from build123d import *

# Parameters (mm, degrees)
ESQUISSE1_R             = 17.5
ESQUISSE1_R_2           = 12.5
BOSS_EXTRU_1_DEPTH      = 65
ESQUISSE3_R             = 2.65
ENL_V_MAT_EXTRU_1_DEPTH = 4
ESQUISSE4_R             = 2
BOSS_EXTRU_2_DEPTH      = 1
BOSS_EXTRU_2_DEPTH_BACK = 2
ENL_V_MAT_EXTRU_2_REACH = 38
ESQUISSE5_R             = 1.05
ENL_V_START             = -3.5
ESQUISSE6_R             = 2.5
ENL_V_MAT_EXTRU_3_DEPTH = 5
CONG_1_R                = 0.5
CHANFREIN1_SIZE         = 0.1
ESQUISSE7_R             = 17.5
BOSS_EXTRU_3_DEPTH      = 5
CHANFREIN2_SIZE         = 2
CHANFREIN3_SIZE         = 1
CHANFREIN3_SIZE2        = 0.577350269


with BuildPart() as part:
    # Esquisse1 → Boss.-Extru.1 (new body, symmetric)
    with BuildSketch(Plane(origin=(0, 0, 0), x_dir=(1, 0, 0), z_dir=(0, 1, 0))):
        Circle(ESQUISSE1_R)
        Circle(ESQUISSE1_R_2, mode=Mode.SUBTRACT)
    extrude(amount=BOSS_EXTRU_1_DEPTH, both=True)

    # Esquisse3 → Enlèv. mat.-Extru.1 (cut)
    with BuildSketch(Plane(origin=(17.5, 0, 0), x_dir=(0, 0, -1), z_dir=(1, 0, 0))):
        Circle(ESQUISSE3_R)
    enl_v_mat_extru_1 = extrude(amount=-ENL_V_MAT_EXTRU_1_DEPTH, mode=Mode.SUBTRACT)

    # Symétrie1: Enlèv. mat.-Extru.1 across plane
    add(enl_v_mat_extru_1.mirror(Plane(origin=(0, 0, 0), x_dir=(0, 0, 1), z_dir=(1, 0, 0))), mode=Mode.SUBTRACT)

    # Esquisse4 → Boss.-Extru.2 (add, two sides)
    with BuildSketch(Plane(origin=(17.5, 0, 0), x_dir=(0, 0, -1), z_dir=(1, 0, 0))) as boss_extru_2_sk:
        with Locations((0, -50)):
            Circle(ESQUISSE4_R)
    extrude(amount=BOSS_EXTRU_2_DEPTH)
    extrude(boss_extru_2_sk.sketch, amount=-BOSS_EXTRU_2_DEPTH_BACK)

    # Esquisse5 → Enlèv. mat.-Extru.2 (cut, up to next)
    with BuildSketch(Plane(origin=(18.5, 0, 0), x_dir=(0, 0, -1), z_dir=(1, 0, 0)), mode=Mode.PRIVATE) as enl_v_mat_extru_2_sk1:
        with Locations((0, -50)):
            Circle(ESQUISSE5_R)
    enl_v_mat_extru_2_tool1 = extrude(enl_v_mat_extru_2_sk1.sketch, amount=-ENL_V_MAT_EXTRU_2_REACH, mode=Mode.PRIVATE) & part.part
    add(enl_v_mat_extru_2_tool1.solids().sort_by_distance((18.5, -50, 0))[0], mode=Mode.SUBTRACT)

    # Esquisse6 → Enlèv. mat.-Extru.3 (cut)
    with BuildSketch(Plane(origin=(18.5, 0, 0), x_dir=(0, 0, -1), z_dir=(1, 0, 0)).offset(ENL_V_START)):
        with Locations((0, -50)):
            Circle(ESQUISSE6_R)
    extrude(amount=-ENL_V_MAT_EXTRU_3_DEPTH, mode=Mode.SUBTRACT)

    # Congé1
    cong_1_edges = [part.edges().sort_by_distance(p)[0] for p in [
        (17.385338651, -50, 2),
    ]]
    fillet(cong_1_edges, radius=CONG_1_R)

    # Chanfrein1
    chanfrein1_edges = [part.edges().sort_by_distance(p)[0] for p in [
        (18.5, -50, 2),
    ]]
    chamfer(chanfrein1_edges, length=CHANFREIN1_SIZE)

    # Esquisse7 → Boss.-Extru.3 (add)
    with BuildSketch(Plane(origin=(0, 65, 0), x_dir=(1, 0, 0), z_dir=(0, 1, 0))):
        Circle(ESQUISSE7_R)
    extrude(amount=-BOSS_EXTRU_3_DEPTH)

    # Chanfrein2
    chanfrein2_edges = [part.edges().sort_by_distance(p)[0] for p in [
        (-17.5, -65, 0),
        (-17.5, 65, 0),
    ]]
    chamfer(chanfrein2_edges, length=CHANFREIN2_SIZE)

    # Chanfrein3
    chanfrein3_edges = [part.edges().sort_by_distance(p)[0] for p in [
        (-12.5, -65, 0),
    ]]
    chanfrein3_side = [part.faces().sort_by_distance(p)[0] for p in [
        (-12.5, -2.5, 0),
    ]]
    chamfer(chanfrein3_edges, length=CHANFREIN3_SIZE, length2=CHANFREIN3_SIZE2, reference=chanfrein3_side[0])


solid = part.part
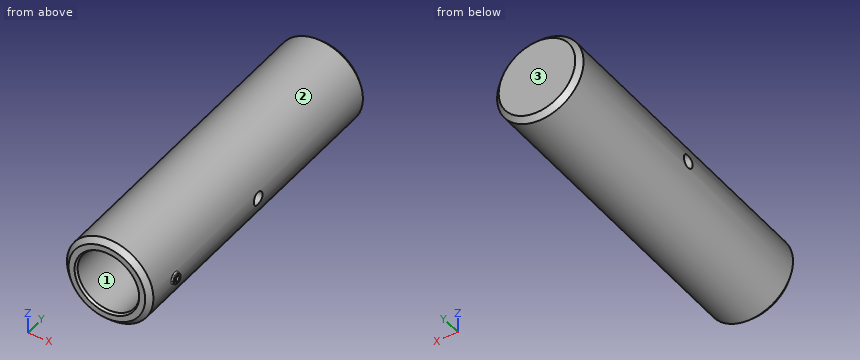
Model file for the job. Use its own axes, mm. Face numbers are marked on the shaded views. Give positions to 0.01 mm unless a question says otherwise; leave off trailing zeros. Write each loop counter-clockwise with the first axis right and the second up, starting at its lowest first coordinate (ties: lowest second). Pieces come first, ordered by that corner, then holes. Notation, with made-up numbers: (-34, 59.25) - (18, 59.25) arc R29 cw to (18, 79.25) - close; hole circle Ø10 at (9.5, 79.5). An arc over 180 degrees is marked (long way). Answer as CSV lines item,"result".
1. Drill centre lines: L1, parallel to Y at x = 14, z = 0; L2, parallel to Y at x = 13.3, z = 0; L3, parallel to Y at x = -15, z = 0. Where is each one in solid material? Low to high. Write a range as [from, to].
Responses:
L1,"y = [-65, -52.5], [-47.5, -2.65], [2.65, 65]"
L2,"y = [-65, -52.5], [-47.5, 65]"
L3,"y = [-65, -2.65], [2.65, 65]"
2. Pin check, flat tips, straight feed: pin 1 (4 mm diameter, centred on x = -0.5, y = -18, fed in from -Z); pin 2 (8 mm diameter, centred on x = 10, y = 24.5, fed in from -Z); pin 3 (3 mm diameter, centred on y = 31.5, z = 11, fed in from -X); pin 4 (4 mm diameter, centred on y = 0, z = 0, fed in from -X). Stop position of each tip, or through.
Responses:
pin 1,"stops at z = -17.5"
pin 2,"stops at z = -16.44"
pin 3,"stops at x = -14.7"
pin 4,"stops at x = -13.5"
3. Band-saw the part on A-A (y = 0). Write the cut outline in (x, z).
Responses:
outline,"(-17.3, -2.65) arc R17.5 ccw to (17.3, -2.65) - (13.5, -2.65) - (13.5, 2.65) - (17.3, 2.65) arc R17.5 ccw to (-17.3, 2.65) - (-13.5, 2.65) - (-13.5, -2.65) - close; hole circle Ø25 at (0, 0)"
4. Band-saw the part on B-B (x = 0). Write the cut outline in (y, z).
Responses:
outline,"(-65, -15.5) - (-63, -17.5) - (63, -17.5) - (65, -15.5) - (65, 15.5) - (63, 17.5) - (-63, 17.5) - (-65, 15.5) - (-65, 13.08) - (-64, 12.5) - (60, 12.5) - (60, -12.5) - (-64, -12.5) - (-65, -13.08) - close"
5. Band-saw the part on C-C (y = -28). Write the cut outline in (x, z).
Responses:
outline,"circle Ø35 at (0, 0); hole circle Ø25 at (0, 0)"
6. Two-plate mould, pull along X, no slides. Class the marked faces 1, 2 and 3: +X half, -X half, draft (parallel to the pull), parting line (faces both ways), or undercut.
Responses:
face 1,"undercut"
face 2,"parting line"
face 3,"draft"
